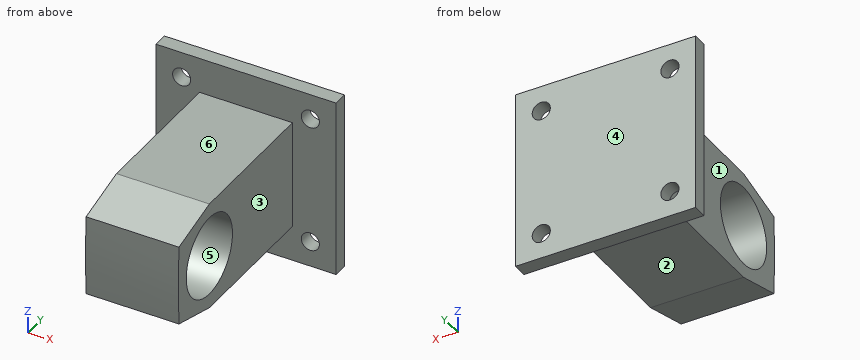
```python
from build123d import *

# Parameters (mm, degrees)
SKETCH1_W           = 32.512
SKETCH1_H           = 38.1
BOSS_EXTRUDE1_DEPTH = 50.292
BOSS_EXTRUDE2_DEPTH = 32.512
SKETCH3_R           = 14
CUT_EXTRUDE1_DEPTH  = 127
SKETCH4_W           = 62.992
SKETCH4_H           = 62.992
BOSS_EXTRUDE3_DEPTH = 5.08
SKETCH5_R           = 3.175
CUT_EXTRUDE2_DEPTH  = 75.105351542


with BuildPart() as part:
    # Sketch1 → Boss-Extrude1 (new body)
    with BuildSketch(Plane(origin=(0, 0, 0), x_dir=(1, 0, 0), z_dir=(0, 1, 0))):
        Rectangle(SKETCH1_W, SKETCH1_H)
    extrude(amount=BOSS_EXTRUDE1_DEPTH)

    # Sketch2 → Boss-Extrude2 (add)
    with BuildSketch(Plane(origin=(16.256, 0, 0), x_dir=(0, 0, -1), z_dir=(1, 0, 0))):
        with BuildLine():
            Line((-19.05, 0), (-14.119497191, -18.400886991))
            ThreePointArc((-14.119497191, -18.400886991), (0, -18.733351542), (14.119497191, -18.400886991))
            Line((14.119497191, -18.400886991), (19.05, 0))
            Line((19.05, 0), (-19.05, 0))
        make_face()
    extrude(amount=-BOSS_EXTRUDE2_DEPTH)

    # Sketch3 → Cut-Extrude1 (cut)
    with BuildSketch(Plane(origin=(16.256, 0, 0), x_dir=(0, 0, -1), z_dir=(1, 0, 0))):
        Circle(SKETCH3_R)
    extrude(amount=-CUT_EXTRUDE1_DEPTH, mode=Mode.SUBTRACT)

    # Sketch4 → Boss-Extrude3 (add)
    with BuildSketch(Plane(origin=(0, 50.292, 0), x_dir=(1, 0, 0), z_dir=(0, 1, 0))):
        Rectangle(SKETCH4_W, SKETCH4_H)
    extrude(amount=BOSS_EXTRUDE3_DEPTH)

    # Sketch5 → Cut-Extrude2 (cut, through all)
    with BuildSketch(Plane(origin=(0, 55.372, 0), x_dir=(1, 0, 0), z_dir=(0, 1, 0))):
        with Locations((-22.515743879, 22.515743879)):
            Circle(SKETCH5_R)
        with Locations((22.515743879, 22.515743879)):
            Circle(SKETCH5_R)
        with Locations((-22.515743879, -22.515743879)):
            Circle(SKETCH5_R)
        with Locations((22.515743879, -22.515743879)):
            Circle(SKETCH5_R)
    extrude(amount=-CUT_EXTRUDE2_DEPTH, mode=Mode.SUBTRACT)


solid = part.part
```
Here's how the part is built. I have some questions about the finished solid (model axes, mm). Face numbers are marked on the shaded views. A direction names the side the tool comes from. Coordinates: 2 decimals unless noted, no trailing zeros. Loops run counter-clockwise (first coordinate to the right, second up) from the corner with the lowest first, then second, coordinate; pieces in that order, holes last. Notation, with made-up numbers: (55, -8) -> (93, -8) arc R9 cw to (93, 3) -> close; hole circle Ø11 at (51, 12). An arc over 180 degrees is marked (long way). Return JSON: item names as keys, results as strings.
1) If we section it at D-D, the plane z = -16: Write out the boundary of the cut face in (x, y).
Results below:
{"outline": "(-31.5, 50.29) -> (-16.26, 50.29) -> (-16.26, -11.38) -> (16.26, -11.38) -> (16.26, 50.29) -> (31.5, 50.29) -> (31.5, 55.37) -> (-31.5, 55.37) -> close"}
2) If we section it at A-A, the plane z = 0: Write out the boundary of the cut face in (x, y).
Results below:
{"outline": "(-31.5, 50.29) -> (-16.26, 50.29) -> (-16.26, 14) -> (16.26, 14) -> (16.26, 50.29) -> (31.5, 50.29) -> (31.5, 55.37) -> (-31.5, 55.37) -> close; (-16.26, -18.73) -> (16.26, -18.73) -> (16.26, -14) -> (-16.26, -14) -> close"}
3) I need wall thicknesses on line 1 (Y direction, x = 19, z = -8); line 2 (X direction, y = 37, z = 19); line 3 (Y direction, x = 14, z = -5). Which ranges of each line are inside material? Lowest first, please. Write a range as from..to.
Results below:
{"line 1": "50.29..55.37", "line 2": "-16.26..16.26", "line 3": "-18.69..-13.08, 13.08..55.37"}
4) Thinking about a two-plate mould opening in Y: for the marked faces 4, 5 and 6, which applies, +Y half, -Y half, draft (parallel to the pull), parting line (faces both ways), or undercut?
Results below:
{"face 4": "+Y half", "face 5": "undercut", "face 6": "draft"}
5) If we section it at B-B, the plane y = -11: Write out the boundary of the cut face in (x, z), then the cut area to 3 significant figures.
Results below:
{"outline": "(-16.26, -16.1) -> (16.26, -16.1) -> (16.26, -8.66) -> (-16.26, -8.66) -> close; (-16.26, 8.66) -> (16.26, 8.66) -> (16.26, 16.1) -> (-16.26, 16.1) -> close", "area": "484 mm²"}
6) Will these pins go through, and if not, where does the flat tip stop? pin 1 (2 mm diameter, centred on x = -12, z = 21, fed in from -Y); pin 2 (2 mm diameter, centred on y = 16.5, z = 10, fed in from +X); pin 3 (8 mm diameter, centred on x = 22.5, y = 10.5, fed in from +Z) (3 decimals); pin 4 (3 mm diameter, centred on x = -6, y = 27.5, fed in from -Z).
Results below:
{"pin 1": "y = 50.29", "pin 2": "x = 16.26", "pin 3": "through", "pin 4": "z = -19.05"}
7) If we section it at C-C, the plane x = -23: Write out the boundary of the cut face in (y, z), then the cut area to 3 significant figures.
Results below:
{"outline": "(50.29, -31.5) -> (55.37, -31.5) -> (55.37, -25.65) -> (50.29, -25.65) -> close; (50.29, -19.38) -> (55.37, -19.38) -> (55.37, 19.38) -> (50.29, 19.38) -> close; (50.29, 25.65) -> (55.37, 25.65) -> (55.37, 31.5) -> (50.29, 31.5) -> close", "area": "256 mm²"}
8) For the marked faces 1, 2 and 3, which set-ups out of +Z, -Z, +X, -X, +Y, -Y let a thin tool reach every point of the face, with its end or its side?
Results below:
{"face 1": "+Z, -Z, -X, -Y", "face 2": "-Z, +X, -X, -Y", "face 3": "+Z, -Z, +X, -Y"}
